from build123d import *

# Parameters (mm, degrees)
SKETCH_R  = 1.6
PAD_DEPTH = 4


with BuildPart() as part:
    # Sketch → Pad (new body)
    with BuildSketch(Plane.XY):
        with BuildLine():
            ThreePointArc((4.35405, 16.458099), (0, 19), (-4.35405, 16.458099))
            Line((-4.35405, 16.458099), (-8, 10))
            Line((-8, 10), (-8, -10))
            Line((-8, -10), (-4.35405, -16.458099))
            ThreePointArc((-4.35405, -16.458099), (0, -19), (4.35405, -16.458099))
            Line((4.35405, -16.458099), (8, -10))
            Line((8, -10), (8, 10))
            Line((8, 10), (4.35405, 16.458099))
        make_face()
        with Locations((0, 14)):
            Circle(SKETCH_R, mode=Mode.SUBTRACT)
        with Locations((0, -14)):
            Circle(SKETCH_R, mode=Mode.SUBTRACT)
    extrude(amount=PAD_DEPTH)


solid = part.part
Build history of the part. All positions in model axes, mm. Round coordinates to 2 decimals unless told otherwise and drop trailing zeros. Loops run counter-clockwise (first coordinate to the right, second up) from the corner with the lowest first, then second, coordinate; pieces in that order, holes last. Notation, with made-up numbers: (26, 49.5) -> (71, 49.5) arc R20 ccw to (71, 87.5) -> close; hole circle Ø5 at (-10, 56). An arc over 180 degrees is marked (long way). Answer in a Markdown table with one row per item.
Item 1: Pin check, flat tips, straight feed: pin 1 (1.5 mm diameter, centred on x = 5.5, z = 0.5, fed in from +Y); pin 2 (4 mm diameter, centred on x = 0, y = 14, fed in from -Z); pin 3 (2 mm diameter, centred on x = -1.5, z = 3.5, fed in from +Y); pin 4 (2.5 mm diameter, centred on x = 0, y = -14, fed in from +Z). Stop position of each tip, or through.
Answers below:
| item | result |
|---|---|
| pin 1 | stops at y = 15.76 |
| pin 2 | stops at z = 0 |
| pin 3 | stops at y = 18.97 |
| pin 4 | passes through |
Item 2: Saw through at B-B (z = 0.6). Write the cut outline in (x, y), and give its area (3 significant figures).
Answers below:
| item | result |
|---|---|
| outline | (-8, -10) -> (-4.35, -16.46) arc R5 ccw to (4.35, -16.46) -> (8, -10) -> (8, 10) -> (4.35, 16.46) arc R5 ccw to (-4.35, 16.46) -> (-8, 10) -> close; hole circle Ø3.2 at (0, -14); hole circle Ø3.2 at (0, 14) |
| area | 495 mm² |
Item 3: Saw through at A-A (x = 0). Write the cut outline in (y, z), and give its area (3 significant figures).
Answers below:
| item | result |
|---|---|
| outline | (-19, 0) -> (-15.6, 0) -> (-15.6, 4) -> (-19, 4) -> close; (-12.4, 0) -> (12.4, 0) -> (12.4, 4) -> (-12.4, 4) -> close; (15.6, 0) -> (19, 0) -> (19, 4) -> (15.6, 4) -> close |
| area | 126 mm² |
Item 4: Saw through at D-D (y = -14.5). Write the cut outline in (x, z).
Answers below:
| item | result |
|---|---|
| outline | (-5.46, 0) -> (-1.52, 0) -> (-1.52, 4) -> (-5.46, 4) -> close; (1.52, 0) -> (5.46, 0) -> (5.46, 4) -> (1.52, 4) -> close |
Item 5: Mould opens along X. For faces 1 (the flat face through (6.203, 13.184, 1.972)), 2 (the cylindrical face through (-0.208, 15.586, 1.972)), 3 (the flat face through (-6.152, 13.274, 1.972)) say: +X half, -X half, draft (parallel to the pull), parting line (faces both ways), or undercut.
Answers below:
| item | result |
|---|---|
| face 1 | +X half |
| face 2 | undercut |
| face 3 | -X half |
Item 6: Saw through at C-C (y = 13). Write the cut outline in (x, z), and give its area (3 significant figures).
Answers below:
| item | result |
|---|---|
| outline | (-6.31, 0) -> (-1.25, 0) -> (-1.25, 4) -> (-6.31, 4) -> close; (1.25, 0) -> (6.31, 0) -> (6.31, 4) -> (1.25, 4) -> close |
| area | 40.5 mm² |
Item 7: Drill centre lines: L1, parallel to Y at x = 0, z = 1.8; L2, parallel to Y at x = -1, z = 1.55; L3, parallel to X at y = 15, z = 2.65. Where is each one in solid material? Low to high. Write a range as [from, to].
Answers below:
| item | result |
|---|---|
| L1 | y = [-19, -15.6], [-12.4, 12.4], [15.6, 19] |
| L2 | y = [-18.9, -15.25], [-12.75, 12.75], [15.25, 18.9] |
| L3 | x = [-5.18, -1.25], [1.25, 5.18] |
